Source: CAD feature listing. Evaluate the final solid. Frame: model axes, mm. A direction names the side the tool comes from. Coordinates: 2 decimals unless noted, no trailing zeros. Write each loop counter-clockwise with the first axis right and the second up, starting at its lowest first coordinate (ties: lowest second). Pieces come first, ordered by that corner, then holes. Notation, with made-up numbers: (-34, 74) - (-27, 74) arc R20 ccw to (-27, 96) - close; hole circle Ø4 at (-12, 63). An arc over 180 degrees is marked (long way). One line per item, written item: value.
from build123d import *

# Parameters (mm, degrees)
F1_DEPTH = 5.05432
F2_W     = 15.6690403819
F2_H     = 21.0551657914
F3_DEPTH = 5.54634


# Not quite as in the source:
# - a feature names something its author has since deleted; it is built from what else it names


with BuildPart() as f1:
    # F0 (on Front) → F1 (new body)
    with BuildSketch(Plane.XZ):
        with BuildLine():
            ThreePointArc((-8.2431294521, 0), (-8.0211144228, -1.9002385587), (-7.3670285487, -3.6981175654))
            ThreePointArc((-7.3670285487, -3.6981175654), (0, -8.2431294521), (7.3670285487, -3.6981175654))
            ThreePointArc((7.3670285487, -3.6981175654), (8.0211144228, -1.9002385587), (8.2431294521, 0))
            Line((8.2431294521, 0), (0, 0))
            Line((0, 0), (-8.2431294521, 0))
        make_face()
        with BuildLine():
            Line((-25.6580412388, -3.6981175654), (-7.3670285487, -3.6981175654))
            ThreePointArc((-7.3670285487, -3.6981175654), (-8.0211144228, -1.9002385587), (-8.2431294521, 0))
            Line((-8.2431294521, 0), (-25.6580412388, 0))
            Line((-25.6580412388, 0), (-25.6580412388, -3.6981175654))
        make_face()
        with BuildLine():
            ThreePointArc((7.3670285487, -3.6981175654), (0, -8.2431294521), (-7.3670285487, -3.6981175654))
            Line((-7.3670285487, -3.6981175654), (-6.4152840294, -35.7396751265))
            ThreePointArc((-6.4152840294, -35.7396751265), (-0.0952885085, -29.131713029), (6.41811349, -35.5491191149))
            ThreePointArc((6.41811349, -35.5491191149), (6.4174060859, -35.6444076234), (6.4152840294, -35.7396751265))
            Line((6.4152840294, -35.7396751265), (7.3670285487, -3.6981175654))
        make_face()
        with BuildLine():
            ThreePointArc((8.2431294521, 0), (8.0211144228, -1.9002385587), (7.3670285487, -3.6981175654))
            Line((7.3670285487, -3.6981175654), (25.6736125353, -3.6981175654))
            Line((25.6736125353, -3.6981175654), (25.6736125353, 0))
            Line((25.6736125353, 0), (8.2431294521, 0))
        make_face()
        with BuildLine():
            ThreePointArc((8.2431294521, 0), (0, 8.2431294521), (-8.2431294521, 0))
            Line((-8.2431294521, 0), (0, 0))
            Line((0, 0), (8.2431294521, 0))
        make_face()
        Polygon((-32.1215167642, -3.9506237954), (-25.6580412388, -3.6981175654), (-25.6580412388, 0), (-32.1215167642, 11.7184091359), align=None)
        with BuildLine():
            ThreePointArc((6.41811349, -35.5491191149), (-0.0952885085, -29.131713029), (-6.4152840294, -35.7396751265))
            ThreePointArc((-6.4152840294, -35.7396751265), (0, -41.9672326049), (6.4152840294, -35.7396751265))
            ThreePointArc((6.4152840294, -35.7396751265), (6.4174060859, -35.6444076234), (6.41811349, -35.5491191149))
        make_face()
        Polygon((25.6736125353, 0), (25.6736125353, -3.6981175654), (32.1235085251, -3.5498465956), (32.1235085251, 12.1219534044), align=None)
    extrude(amount=-F1_DEPTH)

    # F2 (on Front) → F3 (join)
    with BuildSketch(Plane.XZ):
        Polygon((-7.834520191, 64.9923454344), (7.834520191, 64.9923454344), (0, 104.1657105088), align=None)
        with Locations((0, 54.4647625387)):
            Rectangle(F2_W, F2_H)
        Polygon((7.834520191, 4.6665664136), (7.834520191, 26.9957184792), (0, 26.9957184792), (-7.834520191, 26.9957184792), (-7.834520191, 4.6673454344), align=None)
        Polygon((7.834520191, 26.9957184792), (7.834520191, 43.937179643), (-7.834520191, 43.937179643), (-7.834520191, 26.9957184792), (0, 26.9957184792), align=None)
    extrude(amount=-F3_DEPTH)


solid = f1.part
1) Section query B-B on z = 31.5. Output: boundary loops of the cut face in (x, y), then the cut area to 3 significant figures.
Values found:
outline: (-7.83, 0) - (7.83, 0) - (7.83, 5.55) - (-7.83, 5.55) - close
area: 86.9 mm2
2) Material intervals for line 1 (X direction, y = 3.9, z = 6.5); line 2 (X direction, y = 3.25, z = 72); line 3 (Z direction, x = 24, y = 2.4), sorted ascending.
Values found:
line 1: -32.12 to -29.24, -7.83 to 7.83, 29.13 to 32.12
line 2: -6.43 to 6.43
line 3: -3.7 to 0
3) Draft query along Z for faces 4 (the cylindrical face through (-7.86, 2.49, 2.48)), 5 (the flat face through (16, 2, -3.698)), 6 (the flat face through (7.835, 3, 34)), 7 (the cylindrical face through (7.883, 2.492, 2.41)). Return one class per face: released by +Z, released by -Z, zero draft, split by the parting line, or undercut.
Values found:
face 4: undercut
face 5: released by -Z
face 6: zero draft
face 7: undercut
4) Reachability of faces 1 (the flat face through (-3.862, 2.734, 84.853)), 2 (the flat face through (-28.845, 2.492, 5.777)), 3 (the flat face through (-28.935, 2.492, -3.826)) from +Z, -Z, +X, -X, +Y, -Y: full face, straight path, thin tool, end or side. Return the list, or none.
Values found:
face 1: +Z, -X, +Y, -Y
face 2: +Z, +Y, -Y
face 3: -Z, +Y, -Y
5) Contact query for flat-ended pins moving along their axis: P1, Ø3, axis at x = 21, y = 2, coming from the -Z side; P2, Ø1.7, axis at x = -1.5, y = 3.5, coming from the -Z side; P3, Ø1.5, axis at x = -17.5, y = 2.5, coming from the +Z side. Output: stop coordinate, or through.
Values found:
P1: z = -3.7
P2: z = -41.93
P3: z = 0
6) Section query A-A on y = 1.8. Output: boundary loops of the cut face in (x, z).
Values found:
outline: (-32.12, -3.95) - (-25.66, -3.7) - (-7.37, -3.7) - (-6.42, -35.74) arc R6.42 ccw to (6.42, -35.74) - (7.37, -3.7) - (25.67, -3.7) - (32.12, -3.55) - (32.12, 12.12) - (25.67, 0) - (8.24, 0) arc R8.24 ccw to (6.79, 4.67) - (7.83, 4.67) - (7.83, 64.99) - (0, 104.17) - (-7.83, 64.99) - (-7.83, 4.67) - (-6.79, 4.67) arc R8.24 ccw to (-8.24, 0) - (-25.66, 0) - (-32.12, 11.72) - close
7) Section query C-C on z = -14.5. Output: boundary loops of the cut face in (x, y), then the cut area to 3 significant figures.
Values found:
outline: (-7.05, 0) - (7.05, 0) - (7.05, 5.05) - (-7.05, 5.05) - close
area: 71.2 mm2
